Verification items for this drawing (mm, ordinates from the low corner). Round coordinates to 2 decimals unless told otherwise and drop trailing zeros. Write each loop counter-clockwise with the first axis right and the second up, starting at its lowest first coordinate (ties: lowest second). Pieces come first, ordered by that corner, then holes. Notation, with made-up numbers: (3.25, -2) -> (58.25, -2) arc R21 ccw to (58.25, 11) -> close; hole circle Ø9 at (0.5, 70). An arc over 180 degrees is marked (long way). Use one line per item in the form item = value. Start each with the question number.
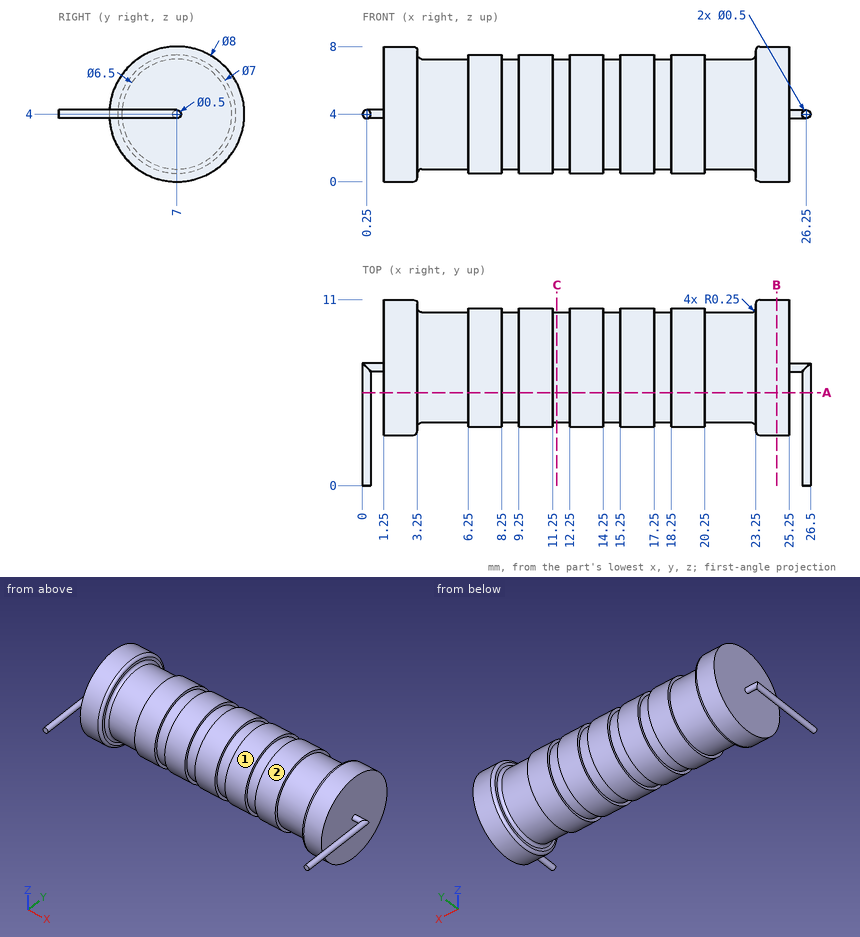
1. Sectioned sample at C-C (x = 11.5). Enter the section's corners in (y, z).
2. Scan lines: probe 1 along X at (y, z) = (9.75, 3.25); probe 2 along Z at (x, y) = (8.75, 7); probe 3 along Y at (x, z) = (6.75, 4.25). Record each from-to range of solid material in increasing order.
3. Sectioned sample at A-A (y = 5.5). Give the number of separate pieces and of enclosed holes in the cut face, and give its area (3 significant figures).
4. Sectioned sample at B-B (x = 24.5). Enter the section's corners in (y, z), and give its area (3 significant figures).
5. Mould release check, pull along X, two halves, no side actions. Record for the marked faces 1 and 2: +X half, -X half, draft (parallel to the pull), parting line (faces both ways), or undercut.
6. Depth check by flat-ended pin: pin 1 (3 mm diameter, centred on y = 5, z = 7, fed in from -X); pin 2 (3 mm diameter, centred on x = 9.5, z = 6.5, fed in from +Y); pin 3 (1 mm diameter, centred on x = 20.5, y = 6.5, fed in from -Z). Enter the tip coordinate at first touch or a pass-through.
Returned:
q1.outline = circle Ø6.5 at (7, 4)
q2.probe_1 = 1.25 to 25.25
q2.probe_2 = 0.75 to 7.25
q2.probe_3 = 3.51 to 10.49
q3.separate_pieces = 3
q3.enclosed_holes = 0
q3.area = 151 mm^2
q4.outline = circle Ø8 at (7, 4)
q4.area = 50.3 mm^2
q5.face_1 = undercut
q5.face_2 = undercut
q6.pin_1 = 1.25
q6.pin_2 = 10.35
q6.pin_3 = 0.5
